```python
from build123d import *

# Parameters (mm, degrees)
F0_R            = 45
F0_W            = 40
F0_H            = 40
F1_DEPTH        = 100
F2_R            = 34
F2_W            = 40
F2_H            = 40
F3_DEPTH        = 25
F4_R            = 37.5
F5_DEPTH        = 80
F5_DEPTH_BACK   = 50
F6_SIZE         = 2
F7_W            = 12
F7_H            = 15
F8_DEPTH        = 80
F8_COPIES_COUNT = 10
F9_SIZE         = 0.5
F10_R           = 27.5
F11_DEPTH       = 35
F12_SIZE        = 2
F13_SIZE        = 1


# Not quite as in the source:
# - a pattern or mirror of a feature is missing from the dataset's text; its kind, count and spacing are read off the source's solid


with BuildPart() as f1:
    # F0 (on Front) → F1 (new body)
    with BuildSketch(Plane.XZ):
        Circle(F0_R)
        Rectangle(F0_W, F0_H, mode=Mode.SUBTRACT)
    extrude(amount=F1_DEPTH)

    # F2 (on face) → F3 (join)
    with BuildSketch(Plane.XZ.offset(100)):
        Circle(F2_R)
        Rectangle(F2_W, F2_H, mode=Mode.SUBTRACT)
    extrude(amount=F3_DEPTH)

    # F4 (on face) → F5 (join, two sides)
    with BuildSketch(Plane(origin=(0, 0, 0), x_dir=(-1, 0, 0), z_dir=(0, 1, 0))) as f5_sk:
        Circle(F4_R)
    extrude(amount=F5_DEPTH)
    extrude(f5_sk.sketch, amount=-F5_DEPTH_BACK)

    # F6
    f6_edges = [f1.edges().sort_by_distance(p)[0] for p in [
        (37.5, 80, 0),
    ]]
    chamfer(f6_edges, length=F6_SIZE)

    # F7 (on face) → F8 (cut, through all)
    with BuildSketch(Plane(origin=(0, 80, 0), x_dir=(-1, 0, 0), z_dir=(0, 1, 0))):
        with Locations((0, 39)):
            Rectangle(F7_W, F7_H)
    f8 = extrude(amount=-F8_DEPTH, mode=Mode.SUBTRACT)

    # F8_copies: F8 ×10 about axis
    f8_copies_axis = Axis((0, 0, 0), (0, 1, 0))
    for i in range(1, F8_COPIES_COUNT):
        add(f8.rotate(f8_copies_axis, i * 360 / F8_COPIES_COUNT), mode=Mode.SUBTRACT)

    # F9
    f9_edges = [f1.edges().sort_by_distance(p)[0] for p in [
        (45, -50, 0),
        (-45, 0, 0),
        (-45, -100, 0),
    ]]
    chamfer(f9_edges, length=F9_SIZE)

    # F10 (on face) → F11 (join)
    with BuildSketch(Plane(origin=(0, 80, 0), x_dir=(-1, 0, 0), z_dir=(0, 1, 0))):
        Circle(F10_R)
    extrude(amount=F11_DEPTH)

    # F12
    f12_edges = [f1.edges().sort_by_distance(p)[0] for p in [
        (27.5, 115, 0),
    ]]
    chamfer(f12_edges, length=F12_SIZE)

    # F13
    f13_edges = [f1.edges().sort_by_distance(p)[0] for p in [
        (-34, -125, 0),
        (0, -125, 20),
        (20, -125, 0),
        (0, -125, -20),
        (-20, -125, 0),
    ]]
    chamfer(f13_edges, length=F13_SIZE)


solid = f1.part
```
CAD build for the part. Positions are in the model's coordinates, mm. A direction names the side the tool comes from. Round coordinates to 2 decimals unless told otherwise and drop trailing zeros. Loops run counter-clockwise (first coordinate to the right, second up) from the corner with the lowest first, then second, coordinate; pieces in that order, holes last. Notation, with made-up numbers: M 46,3.25 L 77,3.25 A25 ccw 77,15.25 Z; hole C 14.5,32.5 d10. An arc over 180 degrees is marked long. Use a Markdown table: item, result. Add a question column.
(1) Which spindle directions (+Z, -Z, +X, -X, +Y, -Y) get a long thin tool onto all of the face, cutting with end or side? Do faces 5 (the face through (-34.4, 40.56, -4.87)), 6 (the face through (30.69, 40.56, 16.28)), 7 (the face through (0, 41, 31.5)), 8 (the face through (-6, 41, -34)), 9 (the face through (11.66, 38.45, -35.64)). Say none if no direction does.
(2) Cut at A-A (y = -70). Give the cut face in (x, z), and give its area (3 significant figures).
(3) Cut at D-D (y = -4). Give the cut face in (x, z).
(4) Flat gauge pins, fed straight in: pin 1 (1.7 mm diameter, centred on y = 55.5, z = -33, fed in from +X); pin 2 (1.5 mm diameter, centred on x = 5, z = 0.5, fed in from -Y); pin 3 (10 mm diameter, centred on x = 24.5, z = -18.5, fed in from +Y). Where does each tip first touch, or does it go through?
(5) Drill centre lines: line 1 (X direction, y = -84.5, z = -2); line 2 (Y direction, x = 3, z = -40); line 3 (Y direction, x = 9.5, z = 26.5). Where is each one in solid material? Low to high.
(6) Pull direction X, two halves, no side cores. Call faces 1 (the face through (30.385, 38.454, -21.977)), 2 (the face through (0, 115, 0)), 3 (the face through (18.583, 40.56, 25.435)), 4 (the face through (-15.26, 40.56, 31.21)): +X half, -X half, draft (parallel to the pull), parting line (faces both ways), or undercut.
Geometry says:
| question | item | result |
|---|---|---|
| 1 | face 5 | +Y |
| 1 | face 6 | +X, +Y |
| 1 | face 7 | +Z, +Y |
| 1 | face 8 | -Z, +Y |
| 1 | face 9 | -Z, +X, +Y |
| 2 | outline | C 0,0 d90; hole M -20,-20 L 20,-20 L 20,20 L -20,20 Z |
| 2 | area | 4,760 mm² |
| 3 | outline | C 0,0 d90 |
| 4 | pin 1 | stops at x = 16.9 |
| 4 | pin 2 | stops at y = -50 |
| 4 | pin 3 | stops at y = 114.8 |
| 5 | line 1 | x = -44.96 to -20, 20 to 44.96 |
| 5 | line 2 | y = -100 to 0 |
| 5 | line 3 | y = -125 to 80 |
| 6 | face 1 | +X half |
| 6 | face 2 | draft |
| 6 | face 3 | undercut |
| 6 | face 4 | -X half |
